Design review of the part built by this model. Coordinates are the model's own, in mm. Round coordinates to 2 decimals unless told otherwise and drop trailing zeros. Write each loop counter-clockwise with the first axis right and the second up, starting at its lowest first coordinate (ties: lowest second). Pieces come first, ordered by that corner, then holes. Notation, with made-up numbers: M -31.75,-8.5 L -24.75,-8.5 A33 ccw -24.75,29.5 Z; hole C 79.5,68 d10. An arc over 180 degrees is marked long. One line per question, with ' | ' between items. Start each with the question number.
Item 1: Add section A-A, the plane y = 0.9. State the section outline as (x, z) points.
Item 2: For L1, parallel to Z at x = 12, y = 1; L2, parallel to X at y = 1.15, z = -5.5; L3, parallel to Z at x = 8, y = 0.35, list the stretches that pass through material, from the lowest coordinate up.
Item 3: Add section B-B, the plane y = 0.15. State the section outline as (x, z) points, and give its area (3 significant figures).
Item 4: Draft analysis for pull direction X (two halves, no side actions). For faces 1 (the face through (1, 1.1, -1)), 2 (the face through (6, 0, -3)), state which applies: released by +X, released by -X, zero draft, split by the parting line, or undercut.
```python
from build123d import *

# Parameters (mm, degrees)
ESQUISSE1_W             = 12.6
ESQUISSE1_H             = 6
BOSS_EXTRU_1_DEPTH      = 1.2
CHANFREIN1_SIZE         = 0.5
CHANFREIN1_SIZE2        = 0.1
CHANFREIN2_SIZE         = 0.1
CHANFREIN2_SIZE2        = 0.5
CHANFREIN3_SIZE         = 0.5
CHANFREIN3_SIZE2        = 0.1
CHANFREIN4_SIZE         = 0.1
CHANFREIN4_SIZE2        = 0.5
CHANFREIN5_SIZE         = 0.5
CHANFREIN5_SIZE2        = 0.1
CHANFREIN6_SIZE         = 0.1
CHANFREIN6_SIZE2        = 0.5
CHANFREIN7_SIZE         = 0.5
CHANFREIN7_SIZE2        = 0.1
CHANFREIN8_SIZE         = 0.1
CHANFREIN8_SIZE2        = 0.5
ESQUISSE2_R             = 0.436243036
ENL_V_MAT_EXTRU_1_DEPTH = 0.1


with BuildPart() as part:
    # Esquisse1 → Boss.-Extru.1 (new body)
    with BuildSketch(Plane(origin=(0, 0, 0), x_dir=(1, 0, 0), z_dir=(0, 1, 0))):
        with Locations((6.3, 3)):
            Rectangle(ESQUISSE1_W, ESQUISSE1_H)
    extrude(amount=BOSS_EXTRU_1_DEPTH)

    # Chanfrein1
    chanfrein1_edges = [part.edges().sort_by_distance(p)[0] for p in [
        (6.3, 1.2, 0),
    ]]
    chanfrein1_side = [part.faces().sort_by_distance(p)[0] for p in [
        (6.3, 0.6, 0),
    ]]
    chamfer(chanfrein1_edges, length=CHANFREIN1_SIZE, length2=CHANFREIN1_SIZE2, reference=chanfrein1_side[0])

    # Chanfrein2
    chanfrein2_edges = [part.edges().sort_by_distance(p)[0] for p in [
        (6.3, 0, 0),
    ]]
    chanfrein2_side = [part.faces().sort_by_distance(p)[0] for p in [
        (6.3, 0, -3),
    ]]
    chamfer(chanfrein2_edges, length=CHANFREIN2_SIZE, length2=CHANFREIN2_SIZE2, reference=chanfrein2_side[0])

    # Chanfrein3
    chanfrein3_edges = [part.edges().sort_by_distance(p)[0] for p in [
        (6.3, 1.2, -6),
    ]]
    chanfrein3_side = [part.faces().sort_by_distance(p)[0] for p in [
        (6.3, 0.6, -6),
    ]]
    chamfer(chanfrein3_edges, length=CHANFREIN3_SIZE, length2=CHANFREIN3_SIZE2, reference=chanfrein3_side[0])

    # Chanfrein4
    chanfrein4_edges = [part.edges().sort_by_distance(p)[0] for p in [
        (6.3, 0, -6),
    ]]
    chanfrein4_side = [part.faces().sort_by_distance(p)[0] for p in [
        (6.3, 0, -3.05),
    ]]
    chamfer(chanfrein4_edges, length=CHANFREIN4_SIZE, length2=CHANFREIN4_SIZE2, reference=chanfrein4_side[0])

    # Chanfrein5
    chanfrein5_edges = [part.edges().sort_by_distance(p)[0] for p in [
        (0, 1.2, -3),
    ]]
    chanfrein5_side = [part.faces().sort_by_distance(p)[0] for p in [
        (0, 0.6, -3),
    ]]
    chamfer(chanfrein5_edges, length=CHANFREIN5_SIZE, length2=CHANFREIN5_SIZE2, reference=chanfrein5_side[0])

    # Chanfrein6
    chanfrein6_edges = [part.edges().sort_by_distance(p)[0] for p in [
        (0, 0, -3),
    ]]
    chanfrein6_side = [part.faces().sort_by_distance(p)[0] for p in [
        (6.3, 0, -3),
    ]]
    chamfer(chanfrein6_edges, length=CHANFREIN6_SIZE, length2=CHANFREIN6_SIZE2, reference=chanfrein6_side[0])

    # Chanfrein7
    chanfrein7_edges = [part.edges().sort_by_distance(p)[0] for p in [
        (12.6, 1.2, -3),
    ]]
    chanfrein7_side = [part.faces().sort_by_distance(p)[0] for p in [
        (12.6, 0.6, -3),
    ]]
    chamfer(chanfrein7_edges, length=CHANFREIN7_SIZE, length2=CHANFREIN7_SIZE2, reference=chanfrein7_side[0])

    # Chanfrein8
    chanfrein8_edges = [part.edges().sort_by_distance(p)[0] for p in [
        (12.6, 0, -3),
    ]]
    chanfrein8_side = [part.faces().sort_by_distance(p)[0] for p in [
        (6.35, 0, -3),
    ]]
    chamfer(chanfrein8_edges, length=CHANFREIN8_SIZE, length2=CHANFREIN8_SIZE2, reference=chanfrein8_side[0])

    # Esquisse2 → Enlèv. mat.-Extru.1 (cut)
    with BuildSketch(Plane(origin=(0, 1.2, 0), x_dir=(-1, 0, 0), z_dir=(0, 1, 0))):
        with Locations(Location((-0.908756143, -0.866244747, 0), (0, 0, 90))):  # turned: the seam where the file's is
            Circle(ESQUISSE2_R)
    extrude(amount=-ENL_V_MAT_EXTRU_1_DEPTH, mode=Mode.SUBTRACT)


solid = part.part
```
Computed values:
1) outline: M 0.04,-5.96 L 12.56,-5.96 L 12.56,-0.04 L 0.04,-0.04 Z
2) L1: z = -5.94 to -0.06 | L2: x = 0.09 to 12.51 | L3: z = -5.97 to -0.03
3) outline: M 0.07,-5.93 L 12.53,-5.93 L 12.53,-0.07 L 0.07,-0.07 Z | area: 73.0 mm^2
4) face 1: undercut | face 2: zero draft
